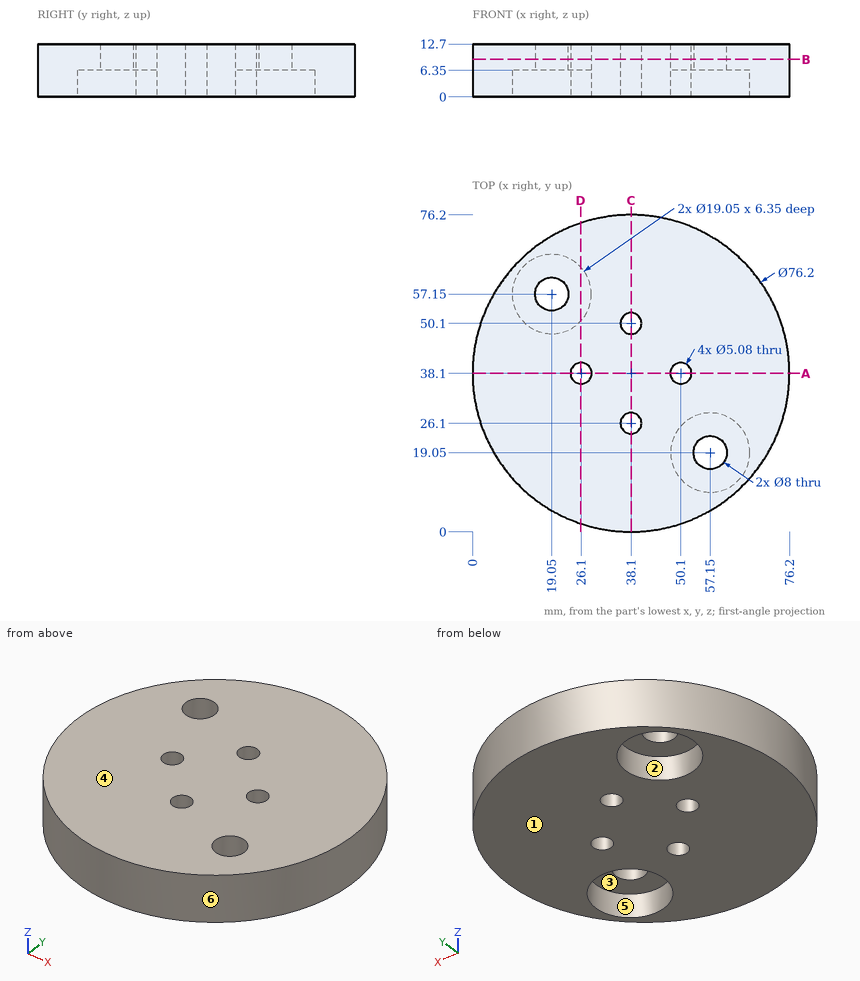
Source: three-view drawing plus pictorial views. Frame: mm from the lowest corner of the part. A direction names the side the tool comes from. Give positions to 0.01 mm unless a question says otherwise; leave off trailing zeros. Write each loop counter-clockwise with the first axis right and the second up, starting at its lowest first coordinate (ties: lowest second). Pieces come first, ordered by that corner, then holes. Notation, with made-up numbers: (84, 80.25) -> (118, 80.25) arc R32 cw to (118, 107.25) -> close; hole circle Ø3 at (4.25, 58). An arc over 180 degrees is marked (long way). Answer in a Markdown table with one row per item.
(1) Section query B-B on z = 9. Return loops of the section in (x, y).
Answers below:
| item | result |
|---|---|
| outline | circle Ø76.2 at (38.1, 38.1); hole circle Ø8 at (19.05, 57.15); hole circle Ø5.08 at (26.1, 38.1); hole circle Ø5.08 at (38.1, 26.1); hole circle Ø5.08 at (38.1, 50.1); hole circle Ø5.08 at (50.1, 38.1); hole circle Ø8 at (57.15, 19.05) |
(2) Pin query (flat end, axial travel): pin 1 (5 mm diameter, centred on y = 17.5, z = 6, fed in from -X); pin 2 (2 mm diameter, centred on y = 24, z = 9.5, fed in from +X); pin 3 (11.5 mm diameter, centred on x = 19.05, y = 57.15, fed in from -Z). Return the tip coordinate at first contact, or that it passes through.
Answers below:
| item | result |
|---|---|
| pin 1 | x = 4.57 |
| pin 2 | x = 73.88 |
| pin 3 | z = 6.35 |
(3) Ray query, line 1 along Y through (x, z) = (38.1, 4.25); line 2 along X through (y, z) = (37, 11.25); line 3 along Y through (x, z) = (36, 0.75). Return the intervals inside material, ascending. Write a range as [from, to].
Answers below:
| item | result |
|---|---|
| line 1 | [0, 23.56], [28.64, 47.56], [52.64, 76.2] |
| line 2 | [0.02, 23.81], [28.39, 47.81], [52.39, 76.18] |
| line 3 | [0.06, 24.67], [27.53, 48.67], [51.53, 76.14] |
(4) Draft query along Y for the marked faces 3, 4, 5 and 6. Return one class per face: +Y half, -Y half, draft (parallel to the pull), parting line (faces both ways), or undercut.
Answers below:
| item | result |
|---|---|
| face 3 | undercut |
| face 4 | draft |
| face 5 | undercut |
| face 6 | parting line |
(5) Set-up query: the marked faces 1 and 2. Return all of +Z, -Z, +X, -X, +Y, -Y with unobstructed straight access to the full face (end or side cutting, diameter ignored); none if empty.
Answers below:
| item | result |
|---|---|
| face 1 | -Z, +X, -X, +Y, -Y |
| face 2 | -Z |
(6) Section query A-A on y = 38.1. Return loops of the section in (x, z), then the cut area to 3 significant figures.
Answers below:
| item | result |
|---|---|
| outline | (0, 0) -> (23.56, 0) -> (23.56, 12.7) -> (0, 12.7) -> close; (28.64, 0) -> (47.56, 0) -> (47.56, 12.7) -> (28.64, 12.7) -> close; (52.64, 0) -> (76.2, 0) -> (76.2, 12.7) -> (52.64, 12.7) -> close |
| area | 839 mm^2 |
(7) Section query D-D on x = 26. Return loops of the section in (y, z).
Answers below:
| item | result |
|---|---|
| outline | (1.97, 0) -> (35.56, 0) -> (35.56, 12.7) -> (1.97, 12.7) -> close; (40.64, 0) -> (50.64, 0) -> (50.64, 6.35) -> (63.66, 6.35) -> (63.66, 0) -> (74.23, 0) -> (74.23, 12.7) -> (40.64, 12.7) -> close |
